Answer from the drawing. Dimensions are ordinates in mm from the lowest x, y and z of the part. A direction names the side the tool comes from. Give positions to 0.01 mm unless a question says otherwise; leave off trailing zeros. Loops run counter-clockwise (first coordinate to the right, second up) from the corner with the lowest first, then second, coordinate; pieces in that order, holes last.
(1) Straight lines are drawn through the part: probe 1 along Y at (x, z) = (42.95, 34); probe 2 along X at (y, z) = (2, 26); probe 3 along X at (y, z) = (15.5, 11.5) (1 decimal). For each, find the intervals that lie inside material, in ascending order.
(2) Each of these flat-tipped pins is pushed along its axis until it touches: P1, Ø3.5, axis at x = 34, z = 26, coming from the +Y side (3 decimals); P2, Ø6, axis at y = 28, z = 34, coming from the -X side (3 decimals); P3, Ø6, axis at y = 8.69, z = 26, coming from the +X side; P4, Ø4, axis at y = 20, z = 37.31, coming from the +X side (1 decimal). Where does it stop, or does it pass through?
(3) Find section A-A, the plane y = 28. State how many separate pieces and enclosed holes the cut face has.
(4) Which of the six approach directions +Z, -Z, +X, -X, +Y, -Y give full straight-line access (tool end or side, diameter ignored) to the marked faces 1 and 2?
(5) Find section C-C, the plane x = 19. Write down the section's boundary in (y, z) (1 decimal), then the cut area to 3 significant figures.
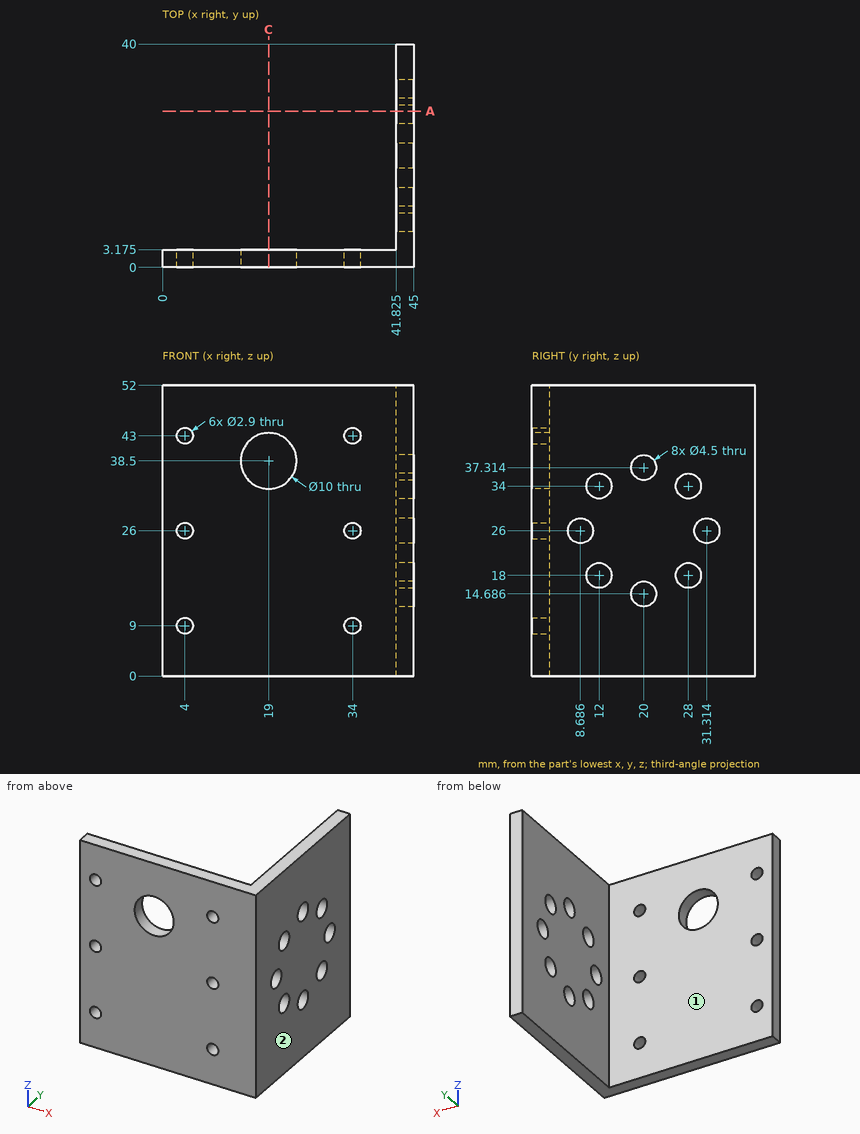
Entries:
1. probe 1: y = 0 to 9.75, 14.25 to 25.75, 30.25 to 40
1. probe 2: x = 0 to 2.55, 5.45 to 32.55, 35.45 to 45
1. probe 3: x = 41.8 to 45
2. P1: stops at y = 3.175
2. P2: stops at x = 41.825
2. P3: stops at x = 45
2. P4: passes through
3. separate pieces: 3
3. enclosed holes: 0
4. face 1: +Z, -Z, -X, +Y
4. face 2: +Z, -Z, +X, +Y, -Y
5. outline: (0, 0) - (3.2, 0) - (3.2, 33.5) - (0, 33.5) - close; (0, 43.5) - (3.2, 43.5) - (3.2, 52) - (0, 52) - close
5. area: 133 mm2
